Verification items for the finished model (mm, model axes). Face numbers are marked on the shaded views. A direction names the side the tool comes from. Coordinates: 2 decimals unless noted, no trailing zeros. Order: outer loops, then holes, each group sorted by start corner. A loop starts at its lowest first (then second) coordinate and runs counter-clockwise, first axis right, second up. Notation, with made-up numbers: M 54.25,9 L 111.25,9 A14 cw 111.25,26 Z; hole C -10.75,-32.75 d9. An arc over 180 degrees is marked long. Return JSON: item names as keys, results as strings. Group by question number.
1. Section check D-D, the plane z = -10.5. Record the cut outline in (x, y).
2. Section check B-B, the plane x = -29.5. Record the cut outline in (y, z) (3 decimals), plus the area to 3 significant figures.
3. Section check A-A, the plane x = 0. Record the cut outline in (y, z), plus the area to 3 significant figures.
4. Section check C-C, the plane y = 7. Record the cut outline in (x, z), plus the area to 3 significant figures.
5. Material ranges on line 1 along Z through (x, y) = (0, 1.5); line 2 along X through (y, z) = (9.5, -5.5); line 3 along Z through (x, y) = (0, 11.7), recorded low to high.
6. Gauge pin test, flat ends, axial feed: pin 1 (1.5 mm diameter, centred on y = 4, z = -9, fed in from -X); pin 2 (1.3 mm diameter, centred on y = 6, z = 1, fed in from -X); pin 3 (6.5 mm diameter, centred on y = 8.5, z = 4, fed in from -X); pin 4 (8 mm diameter, centred on x = 0, z = 0, fed in from -Y). Record the tip position at first contact, or that the pin passes through.
7. Mould release check, pull along Z, two halves, no side actions. Record for the marked faces 4, 5, 6 and 7: +Z half, -Z half, draft (parallel to the pull), parting line (faces both ways), or undercut.
8. Set-up check for the marked faces 1, 2 and 3: record each of +Z, -Z, +X, -X, +Y, -Y from which the full face is reachable in a straight line by a thin tool's end or side.
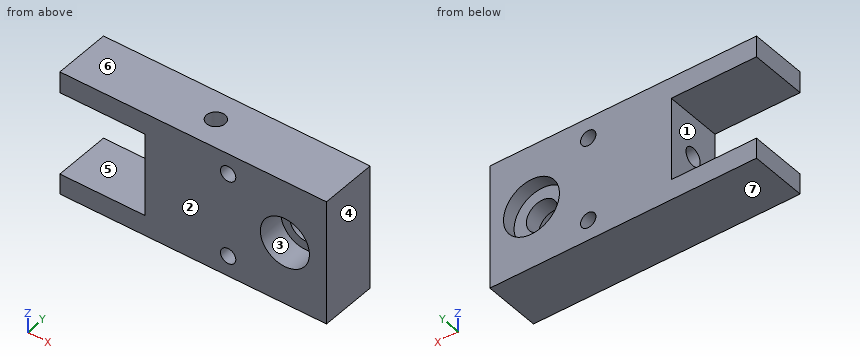
```python
from build123d import *

# Parameters (mm, degrees)
SKETCH1_R              = 3.56
BOSS_EXTRUDE1_DEPTH    = 12.86
SKETCH2_R              = 2.085
CUT_EXTRUDE1_DEPTH     = 12.7
SKETCH3_R              = 6.35
CUT_EXTRUDE2_DEPTH     = 3.12
SKETCH4_R              = 5.57
CUT_EXTRUDE3_DEPTH     = 6.08
SKETCH5_R              = 1.74
CUT_EXTRUDE4_DEPTH     = 13.86
SKETCH6_R              = 1.735
CUT_EXTRUDE_8_32_DEPTH = 5
SKETCH7_R              = 2.1
CUT_EXTRUDE5_DEPTH     = 10


with BuildPart() as part:
    # Sketch1 → Boss-Extrude1 (new body)
    with BuildSketch(Plane(origin=(0, 0, 0), x_dir=(1, 0, 0), z_dir=(0, 1, 0))):
        Polygon((-31.72, 9.53), (-31.72, -9.36), (-51.06, -9.36), (-51.06, -14.18), (9.44, -14.18), (9.44, 14.18), (-51.06, 14.18), (-51.06, 9.53), align=None)
        Circle(SKETCH1_R, mode=Mode.SUBTRACT)
    extrude(amount=BOSS_EXTRUDE1_DEPTH)

    # Sketch2 → Cut-Extrude1 (cut)
    with BuildSketch(Plane.ZY.offset(31.72)):
        with Locations((-0.085, 6.43)):
            Circle(SKETCH2_R)
    extrude(amount=-CUT_EXTRUDE1_DEPTH, mode=Mode.SUBTRACT)

    # Sketch3 → Cut-Extrude2 (cut)
    with BuildSketch(Plane(origin=(0, 12.86, 0), x_dir=(-1, 0, 0), z_dir=(0, 1, 0))):
        Circle(SKETCH3_R)
    extrude(amount=-CUT_EXTRUDE2_DEPTH, mode=Mode.SUBTRACT)

    # Sketch4 → Cut-Extrude3 (cut)
    with BuildSketch(Plane.XZ):
        Circle(SKETCH4_R)
    extrude(amount=-CUT_EXTRUDE3_DEPTH, mode=Mode.SUBTRACT)

    # Sketch5 → Cut-Extrude4 (cut, through all)
    with BuildSketch(Plane.XZ):
        with Locations((-12.88, -9.53)):
            Circle(SKETCH5_R)
        with Locations((-12.88, 9.53)):
            Circle(SKETCH5_R)
    extrude(amount=-CUT_EXTRUDE4_DEPTH, mode=Mode.SUBTRACT)

    # Sketch6 → Cut-Extrude 8-32 (cut)
    with BuildSketch(Plane.XY.offset(14.18)):
        with Locations((-20.615, 6.43)):
            Circle(SKETCH6_R)
    extrude(amount=-CUT_EXTRUDE_8_32_DEPTH, mode=Mode.SUBTRACT)

    # Sketch7 → Cut-Extrude5 (cut)
    with BuildSketch(Plane.XY.offset(14.18)):
        with Locations((-20.615, 6.43)):
            Circle(SKETCH7_R)
    extrude(amount=-CUT_EXTRUDE5_DEPTH, mode=Mode.SUBTRACT)


solid = part.part
```
Answers follow:
{
 "1": {"outline": "M -51.06,0 L -14.32,0 L -14.32,12.86 L -51.06,12.86 Z; M -11.44,0 L 9.44,0 L 9.44,12.86 L -11.44,12.86 Z"},
 "2": {"outline": "M 0,-14.18 L 12.86,-14.18 L 12.86,14.18 L 0,14.18 Z; hole C 6.43,-0.085 d4.17", "area": "351 mm^2"},
 "3": {"outline": "M 0,-14.18 L 12.86,-14.18 L 12.86,-6.35 L 9.74,-6.35 L 9.74,-3.56 L 6.08,-3.56 L 6.08,-5.57 L 0,-5.57 Z; M 0,5.57 L 6.08,5.57 L 6.08,3.56 L 9.74,3.56 L 9.74,6.35 L 12.86,6.35 L 12.86,14.18 L 0,14.18 Z", "area": "231 mm^2"},
 "4": {"outline": "M -51.06,-14.18 L 9.44,-14.18 L 9.44,14.18 L -18.59,14.18 L -18.59,4.18 L -22.64,4.18 L -22.64,14.18 L -51.06,14.18 L -51.06,9.36 L -31.72,9.36 L -31.72,1.92 L -19.02,1.92 L -19.02,-2.09 L -31.72,-2.09 L -31.72,-9.53 L -51.06,-9.53 Z; hole C -12.88,-9.53 d3.48; hole C -12.88,9.53 d3.48; hole C 0,0 d7.12", "area": "1,200 mm^2"},
 "5": {"line 1": "-14.18 to -5.57, 5.57 to 14.18", "line 2": "-31.72 to 9.44", "line 3": "-14.18 to -6.35, 6.35 to 14.18"},
 "6": {"pin 1": "x = -51.06", "pin 2": "x = -19.02", "pin 3": "x = -31.72", "pin 4": "y = 6.08"},
 "7": {"face 4": "draft", "face 5": "undercut", "face 6": "+Z half", "face 7": "-Z half"},
 "8": {"face 1": "-X, +Y, -Y", "face 2": "+Z, -Z, +X, -X, -Y", "face 3": "-Y"}
}
